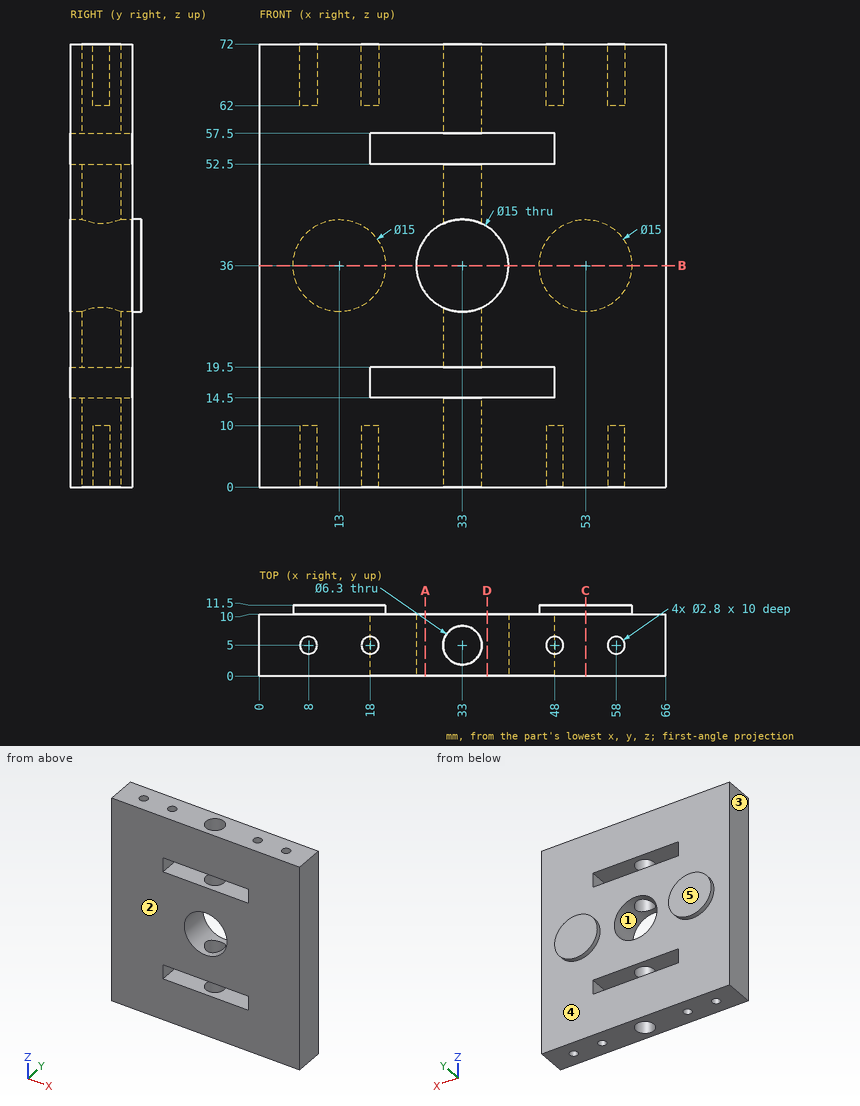
Geometry check sheet. Reference: drawing and pictorial views, mm from the part's lowest x, y, z. A direction names the side the tool comes from. Coordinates: 2 decimals unless noted, no trailing zeros. Loops run counter-clockwise (first coordinate to the right, second up) from the corner with the lowest first, then second, coordinate; pieces in that order, holes last. Notation, with made-up numbers: M -3.5,28.25 L 30.5,28.25 A30 ccw 30.5,65.25 Z; hole C 83,18 d4. An arc over 180 degrees is marked long. One line per item, written item: value.
1. Material ranges on line 1 along Z through (x, y) = (44, 7); line 2 along Y through (x, z) = (33, 69); line 3 along Y through (x, z) = (8, 5), recorded low to high. Write a range as from..to.
Answers follow:
line 1: 0..14.5, 19.5..52.5, 57.5..72
line 2: 0..1.85, 8.15..10
line 3: 0..3.6, 6.4..10
2. Section check B-B on z = 36. Record the cut outline in (x, y).
Answers follow:
outline: M 0,0 L 25.5,0 L 25.5,10 L 20.5,10 L 20.5,11.5 L 5.5,11.5 L 5.5,10 L 0,10 Z; M 40.5,0 L 66,0 L 66,10 L 60.5,10 L 60.5,11.5 L 45.5,11.5 L 45.5,10 L 40.5,10 Z
3. Set-up check for the marked faces 4 and 5: record each of +Z, -Z, +X, -X, +Y, -Y from which the full face is reachable in a straight line by a thin tool's end or side.
Answers follow:
face 4: +Y
face 5: +Z, -Z, +X, -X, +Y
4. Mould release check, pull along X, two halves, no side actions. Record for the marked faces 1, 2 and 3: pulls with the +X half, pulls with the -X half, needs draft (parallel to the pull), parting line crosses it, or undercut.
Answers follow:
face 1: undercut
face 2: needs draft
face 3: pulls with the -X half
5. Gauge pin test, flat ends, axial feed: P1, Ø5, axis at x = 33, y = 5, coming from the -Z side; P2, Ø2, axis at x = 58, y = 5, coming from the +Z side; P3, Ø1.7, axis at x = 48, y = 5, coming from the -Z side; P4, Ø8, axis at x = 9, z = 17, coming from the +Y side. Record the tip position at first contact, or that the pin passes through.
Answers follow:
P1: through
P2: z = 62
P3: z = 10
P4: y = 10
6. Section check A-A on x = 27. Record the cut outline in (y, z).
Answers follow:
outline: M 0,0 L 10,0 L 10,14.5 L 0,14.5 Z; M 0,19.5 L 10,19.5 L 10,31.5 L 0,31.5 Z; M 0,40.5 L 10,40.5 L 10,52.5 L 0,52.5 Z; M 0,57.5 L 10,57.5 L 10,72 L 0,72 Z
7. Section check C-C on x = 53. Record the cut outline in (y, z), plus the area to 4 significant figures.
Answers follow:
outline: M 0,0 L 10,0 L 10,28.5 L 11.5,28.5 L 11.5,43.5 L 10,43.5 L 10,72 L 0,72 Z
area: 742.5 mm^2
8. Section check D-D on x = 37. Record the cut outline in (y, z), plus the area to 3 significant figures.
Answers follow:
outline: M 0,0 L 10,0 L 10,14.5 L 0,14.5 Z; M 0,19.5 L 10,19.5 L 10,29.66 L 0,29.66 Z; M 0,42.34 L 10,42.34 L 10,52.5 L 0,52.5 Z; M 0,57.5 L 10,57.5 L 10,72 L 0,72 Z
area: 493 mm^2
